Geometry check sheet. Reference: the model listing, model coordinates, mm. A direction names the side the tool comes from. Round coordinates to 2 decimals unless told otherwise and drop trailing zeros. Write each loop counter-clockwise with the first axis right and the second up, starting at its lowest first coordinate (ties: lowest second). Pieces come first, ordered by that corner, then holes. Notation, with made-up numbers: M -22,82.5 L 33,82.5 A18 cw 33,116.5 Z; hole C 56.25,86.25 d1. An arc over 180 degrees is marked long. Answer in a Markdown table with one row per item. Add a question column.
from build123d import *

# Parameters (mm, degrees)
F0_R     = 5.2865279156
F1_DEPTH = 25
F2_R     = 39.9170706603
F2_R_2   = 34.6011659379
F3_DEPTH = 75
F4_R     = 11.7194622097
F5_DEPTH = 25
F6_R     = 7.873360038
F6_R_2   = 5.2865279156
F7_DEPTH = 10
F8_R     = 13.6780275644
F8_R_2   = 11.7194622097
F9_DEPTH = 5


with BuildPart() as f1:
    # F0 (on Front) → F1 (new body)
    with BuildSketch(Plane.XZ):
        with BuildLine():
            Line((-10.6633168949, 63.7640005702), (-10.6633168949, 44.8946944847))
            ThreePointArc((-10.6633168949, 44.8946944847), (-40.2070284925, 22.6414394393), (-43.917693949, -14.1589575281))
            Line((-43.917693949, -14.1589575281), (-60.0696593727, -23.4842991134))
            ThreePointArc((-60.0696593727, -23.4842991134), (-66.2598598239, -38.8131493377), (-49.8895858933, -41.1167036046))
            Line((-49.8895858933, -41.1167036046), (-33.5482874715, -31.6820505619))
            ThreePointArc((-33.5482874715, -31.6820505619), (0.4954525136, -46.1410278048), (34.2208638849, -30.9543598714))
            Line((34.2208638849, -30.9543598714), (50.3728293087, -40.2797014568))
            ThreePointArc((50.3728293087, -40.2797014568), (66.7431032393, -37.9761471898), (60.5529027881, -22.6472969656))
            Line((60.5529027881, -22.6472969656), (44.2116043663, -13.2126439228))
            ThreePointArc((44.2116043663, -13.2126439228), (39.7115759789, 23.4995883656), (9.6968300641, 45.1133173995))
            Line((9.6968300641, 45.1133173995), (9.6968300641, 63.7640005702))
            ThreePointArc((9.6968300641, 63.7640005702), (-0.4832434154, 76.7892965276), (-10.6633168949, 63.7640005702))
        make_face()
        with Locations((-57.1745378733, -33.5677362638)):
            Circle(F0_R, mode=Mode.SUBTRACT)
        with Locations((57.6577812887, -32.730734116)):
            Circle(F0_R, mode=Mode.SUBTRACT)
        with Locations((-0.4832434154, 66.2984703798)):
            Circle(F0_R, mode=Mode.SUBTRACT)
    extrude(amount=F1_DEPTH)

    # F2 (on Front) → F3 (join)
    with BuildSketch(Plane.XZ):
        Circle(F2_R)
        Circle(F2_R_2, mode=Mode.SUBTRACT)
    extrude(amount=F3_DEPTH)

    # F4 (on Front) → F5 (cut)
    with BuildSketch(Plane.XZ):
        Circle(F4_R)
    extrude(amount=F5_DEPTH, mode=Mode.SUBTRACT)

    # F6 (on face) → F7 (cut)
    with BuildSketch(Plane.XZ.offset(25)):
        with Locations((-0.4832434154, 66.2984703798)):
            Circle(F6_R)
        with Locations((-0.4832434154, 66.2984703798)):
            Circle(F6_R_2, mode=Mode.SUBTRACT)
        with Locations((-57.1745378733, -33.5677362638)):
            Circle(F6_R)
        with Locations((-57.1745378733, -33.5677362638)):
            Circle(F6_R_2, mode=Mode.SUBTRACT)
        with Locations((57.6577812887, -32.730734116)):
            Circle(F6_R)
        with Locations((57.6577812887, -32.730734116)):
            Circle(F6_R_2, mode=Mode.SUBTRACT)
    extrude(amount=-F7_DEPTH, mode=Mode.SUBTRACT)

    # F8 (on face) → F9 (join)
    with BuildSketch(Plane.XZ.offset(25)):
        Circle(F8_R)
        Circle(F8_R_2, mode=Mode.SUBTRACT)
    extrude(amount=F9_DEPTH)


solid = f1.part
Item 1: Scan lines: probe 1 along X at (y, z) = (-45, 0); probe 2 along Z at (x, y) = (0, -13.75); probe 3 along X at (y, z) = (-14.5, 54). Record each from-to range of solid material in increasing order. Write a range as from..to.
Item 2: Section check A-A, the plane z = 0. Record the boundary of the cut face in (x, y), and give its area (3 significant figures).
Item 3: Section check C-C, the plane y = -23. Record the boundary of the cut face in (x, z), and give its area (3 significant figures).
Item 4: Access from +Z, -Z, +X, -X, +Y, -Y to the whole of each face (thin tool, end or side, straight path). Record for faces 1 (the flat face through (-12, -75, 33)), 2 (the cylindrical face through (-58.2, -20.07, -25.76)), 3 (the flat face through (-41.833, -12.325, -36.465)).
Item 5: Mould release check, pull along Z, two halves, no side actions. Record for faces 4 (the cylindrical face through (-0.037, -12.325, -46.144)), 5 (the flat face through (-10.663, -12, 54)), 6 (the flat face through (14, 0, 3)): +Z half, -Z half, draft (parallel to the pull), parting line (faces both ways), or undercut.
Item 6: Gauge pin test, flat ends, axial feed: pin 1 Ø6 at (y, z) = (-52.5, -9) entering from -X; pin 2 Ø17.5 at (x, z) = (61.5, -33) entering from -Y; pin 3 Ø3 at (x, y) = (-8.5, -21) entering from -Z. Record the tip position at first contact, or that the pin passes through.
Item 7: Section check D-D, the plane x = 17. Record the boundary of the cut face in (y, z).
Item 8: Section check B-B, the plane x = 0. Record the boundary of the cut face in (y, z), and give its area (3 significant figures).
Result sheet:
| question | item | result |
|---|---|---|
| 1 | probe 1 | x = -39.92..-34.6, 34.6..39.92 |
| 1 | probe 2 | z = -46.14..-11.72, 11.72..61.03, 71.56..76.78 |
| 1 | probe 3 | x = -10.66..9.7 |
| 2 | outline | M -46.14,-25 L -39.92,-25 L -39.92,-75 L -34.6,-75 L -34.6,-25 L -13.68,-25 L -13.68,-30 L -11.72,-30 L -11.72,0 L -46.14,0 Z; M 11.72,-30 L 13.68,-30 L 13.68,-25 L 34.6,-25 L 34.6,-75 L 39.92,-75 L 39.92,-25 L 46.14,-25 L 46.14,0 L 11.72,0 Z |
| 2 | area | 2,270 mm^2 |
| 3 | outline | M -60.07,-23.48 A10.49 ccw long -49.89,-41.12 L -33.55,-31.68 A46.14 ccw 34.22,-30.95 L 50.37,-40.28 A10.49 ccw long 60.55,-22.65 L 44.21,-13.21 A46.14 ccw 9.7,45.11 L 9.7,63.76 A10.49 ccw long -10.66,63.76 L -10.66,44.89 A46.14 ccw -43.92,-14.16 Z; hole C -57.17,-33.57 d15.75; hole C 0,0 d23.44; hole C -0.48,66.3 d15.75; hole C 57.66,-32.73 d15.75 |
| 3 | area | 7,450 mm^2 |
| 4 | face 1 | +Z, -Z, +X, -X, -Y |
| 4 | face 2 | -Y |
| 4 | face 3 | -Z, +Y, -Y |
| 5 | face 4 | -Z half |
| 5 | face 5 | undercut |
| 5 | face 6 | draft |
| 6 | pin 1 | stops at x = -39.46 |
| 6 | pin 2 | stops at y = -25 |
| 6 | pin 3 | stops at z = -45.61 |
| 7 | outline | M -75,-36.12 L -25,-36.12 L -25,-42.9 L 0,-42.9 L 0,42.9 L -25,42.9 L -25,36.12 L -75,36.12 L -75,30.14 L -25,30.14 L -25,-30.14 L -75,-30.14 Z |
| 8 | outline | M -75,-39.92 L -25,-39.92 L -25,-46.14 L 0,-46.14 L 0,-11.72 L -30,-11.72 L -30,-13.68 L -25,-13.68 L -25,-34.6 L -75,-34.6 Z; M -75,34.6 L -25,34.6 L -25,13.68 L -30,13.68 L -30,11.72 L 0,11.72 L 0,61.03 L -15,61.03 L -15,58.44 L -25,58.44 L -25,39.92 L -75,39.92 Z; M -25,74.16 L -15,74.16 L -15,71.56 L 0,71.56 L 0,76.78 L -25,76.78 Z |
| 8 | area | 2,720 mm^2 |
